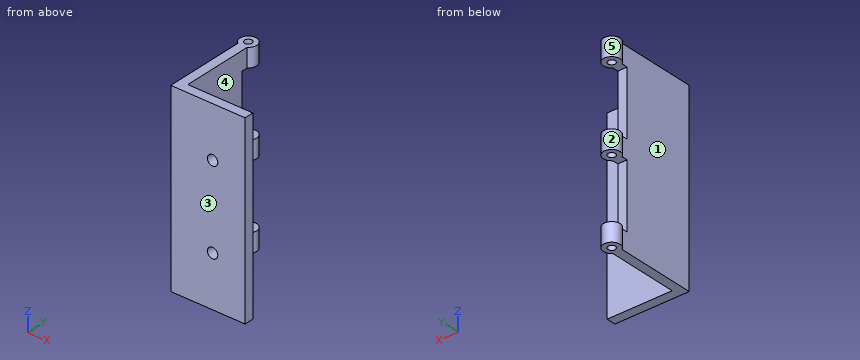
```python
from build123d import *

# Parameters (mm, degrees)
BOSS_EXTRUDE1_DEPTH = 50
SKETCH7_R           = 4.5
SKETCH7_R_2         = 2
SKETCH7_W           = 5
SKETCH7_H           = 3.258342613
BOSS_EXTRUDE4_DEPTH = 5
SKETCH2_R           = 4.5
SKETCH2_R_2         = 2
SKETCH2_W           = 5
SKETCH2_H           = 3.258342613
BOSS_EXTRUDE3_DEPTH = 10
SKETCH12_R          = 2.8
CUT_EXTRUDE1_DEPTH  = 6


with BuildPart() as part:
    # Sketch1 → Boss-Extrude1 (new body, symmetric)
    with BuildSketch(Plane.XY):
        Polygon((0, 0), (0, 40), (5, 40), (5, 5), (40, 5), (40, 0), align=None)
    extrude(amount=BOSS_EXTRUDE1_DEPTH, both=True)

    # Sketch7 → Boss-Extrude4 (add, symmetric)
    with BuildSketch(Plane.XY):
        with Locations((2.5, 47)):
            Circle(SKETCH7_R)
        with Locations((2.5, 47)):
            Circle(SKETCH7_R_2, mode=Mode.SUBTRACT)
        with Locations((2.5, 41.629171306)):
            Rectangle(SKETCH7_W, SKETCH7_H)
    extrude(amount=BOSS_EXTRUDE4_DEPTH, both=True)

    # Sketch2 → Boss-Extrude3 (add)
    with BuildSketch(Plane.XY.offset(50)):
        with Locations((2.5, 47)):
            Circle(SKETCH2_R)
        with Locations((2.5, 47)):
            Circle(SKETCH2_R_2, mode=Mode.SUBTRACT)
        with Locations((2.5, 41.629171306)):
            Rectangle(SKETCH2_W, SKETCH2_H)
    boss_extrude3 = extrude(amount=-BOSS_EXTRUDE3_DEPTH)

    # Mirror1: Boss-Extrude3 across plane
    add(boss_extrude3.mirror(Plane.XY))

    # Sketch12 → Cut-Extrude1 (cut, through all)
    with BuildSketch(Plane(origin=(0, 5, 0), x_dir=(1, 0, 0), z_dir=(0, 1, 0))):
        with Locations((22.5, 22.5)):
            Circle(SKETCH12_R)
        with Locations((22.5, -22.5)):
            Circle(SKETCH12_R)
    extrude(amount=-CUT_EXTRUDE1_DEPTH, mode=Mode.SUBTRACT)


solid = part.part
```
Can you work these out from the model? Positions are in its coordinate system, mm. Face numbers are marked on the shaded views. A direction names the side the tool comes from. Give positions to 0.01 mm unless a question says otherwise; leave off trailing zeros. Loops run counter-clockwise (first coordinate to the right, second up) from the corner with the lowest first, then second, coordinate; pieces in that order, holes last. Notation, with made-up numbers: M 60.5,-14 L 106.5,-14 A8 ccw 106.5,-3 Z; hole C -33,-25 d2. An arc over 180 degrees is marked long. Answer in a Markdown table with one row per item.
1. Which directions (+Z, -Z, +X, -X, +Y, -Y) give clear straight access to the entire face, cutting with the end or side of a thin tool? Please do the marked faces 4 and 5.
Taken from the geometry:
| item | result |
|---|---|
| face 4 | +Z, -Z, +X |
| face 5 | +Z, -Z |
2. Suppose I cut it at A-A on x = 22.5. Write out the boundary of the cut face in (y, z), plus the area to 3 significant figures.
Taken from the geometry:
| item | result |
|---|---|
| outline | M 0,-50 L 5,-50 L 5,-25.3 L 0,-25.3 Z; M 0,-19.7 L 5,-19.7 L 5,19.7 L 0,19.7 Z; M 0,25.3 L 5,25.3 L 5,50 L 0,50 Z |
| area | 444 mm² |
3. Suppose I cut it at B-B on z = -22.5. Write out the boundary of the cut face in (x, y).
Taken from the geometry:
| item | result |
|---|---|
| outline | M 0,0 L 19.7,0 L 19.7,5 L 5,5 L 5,40 L 0,40 Z; M 25.3,0 L 40,0 L 40,5 L 25.3,5 Z |
4. If I drill on line 1 along Z through (x, y) = (22.5, 1.2); line 2 along Y through (x, z) = (2.5, -42.75); line 3 along X through (y, z) = (3.35, 22.5), over which ranges is the centre line in solid material (lowest first)?
Taken from the geometry:
| item | result |
|---|---|
| line 1 | z = -50 to -25.3, -19.7 to 19.7, 25.3 to 50 |
| line 2 | y = 0 to 45, 49 to 51.5 |
| line 3 | x = 0 to 19.7, 25.3 to 40 |
5. Suppose I cut it at D-D on x = 2.5. Write out the boundary of the cut face in (y, z).
Taken from the geometry:
| item | result |
|---|---|
| outline | M 0,-50 L 45,-50 L 45,-40 L 40,-40 L 40,-5 L 45,-5 L 45,5 L 40,5 L 40,40 L 45,40 L 45,50 L 0,50 Z; M 49,-50 L 51.5,-50 L 51.5,-40 L 49,-40 Z; M 49,-5 L 51.5,-5 L 51.5,5 L 49,5 Z; M 49,40 L 51.5,40 L 51.5,50 L 49,50 Z |
6. Suppose I cut it at C-C on y = 47. Write out the boundary of the cut face in (x, z), plus the area to 3 significant figures.
Taken from the geometry:
| item | result |
|---|---|
| outline | M -2,-50 L 0.5,-50 L 0.5,-40 L -2,-40 Z; M -2,-5 L 0.5,-5 L 0.5,5 L -2,5 Z; M -2,40 L 0.5,40 L 0.5,50 L -2,50 Z; M 4.5,-50 L 7,-50 L 7,-40 L 4.5,-40 Z; M 4.5,-5 L 7,-5 L 7,5 L 4.5,5 Z; M 4.5,40 L 7,40 L 7,50 L 4.5,50 Z |
| area | 150 mm² |
7. Thinking about a two-plate mould opening in Y: for the marked faces 1, 2 and 3, which applies, released by +Y, released by -Y, zero draft, split by the parting line, or undercut?
Taken from the geometry:
| item | result |
|---|---|
| face 1 | zero draft |
| face 2 | undercut |
| face 3 | released by -Y |
8. For pin 1 Ø3 at (x, y) = (2.5, 47) entering from +Z; pin 2 Ø6.5 at (x, z) = (22.5, -22.5) entering from -Y; pin 3 Ø3 at (x, z) = (11.5, -39.5) entering from +Y; pin 4 Ø3 at (y, z) = (30, -27) entering from -X, each with a flat end and sliding along its axis, tell me the tip position at first contact or that it passes through.
Taken from the geometry:
| item | result |
|---|---|
| pin 1 | passes through |
| pin 2 | stops at y = 0 |
| pin 3 | stops at y = 5 |
| pin 4 | stops at x = 0 |
